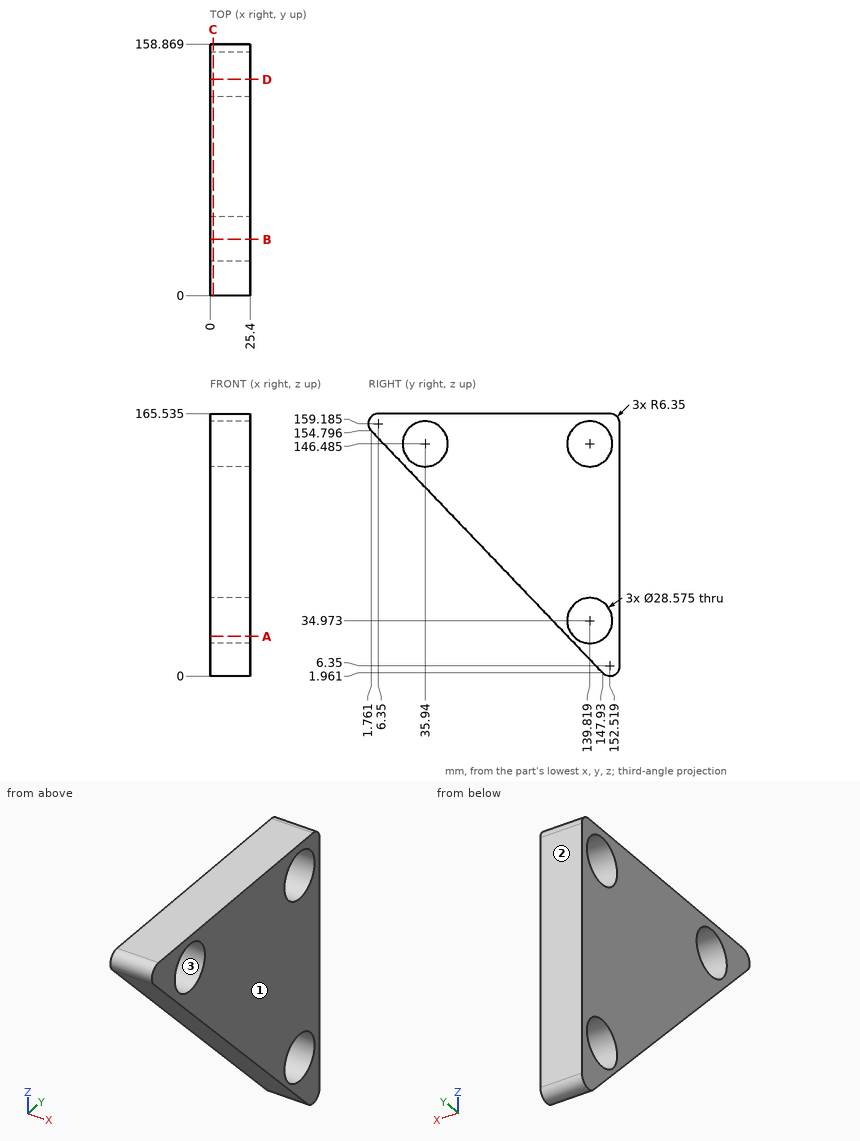
Geometry: see drawing. Coordinates: mm, zero at the bounding-box minimum. Round coordinates to 2 decimals unless told otherwise and drop trailing zeros. Write each loop counter-clockwise with the first axis right and the second up, starting at its lowest first coordinate (ties: lowest second). Pieces come first, ordered by that corner, then holes. Notation, with made-up numbers: M 48,73 L 97,73 A26 cw 97,97 Z; hole C 32.5,57.5 d10. An arc over 180 degrees is marked long. Answer as a JSON object with one key per item and string values. Group by question number.
(1) Section query B-B on y = 35.5. Output: boundary loops of the cut face in (x, z) (1 decimal), then the cut area to 3 significant figures.
(2) First-contact query: pin 1 (4 mm diameter, centred on x = 6.5, z = 50, fed in from -Y) (1 decimal); pin 2 (3 mm diameter, centred on x = 21.5, z = 148, fed in from -Y) (1 decimal); pin 3 (1 mm diameter, centred on x = 20.5, z = 30, fed in from -Y) (1 decimal). Flat tips, straight axial feed; report the tip coordinate or a pass-through.
(3) Section query A-A on z = 25. Output: boundary loops of the cut face in (x, y), then the cut area to 3 significant figures.
(4) Section query D-D on y = 136.5. Output: boundary loops of the cut face in (x, z) (1 decimal).
(5) Section query C-C on x = 2. State how many separate pieces and enclosed holes the cut face has, then the cut area to 3 significant figures.
(6) Mould query, pull axis Y, two halves, no side actions, for the marked faces 1, 2 and 3. Classes: +Y half, -Y half, draft (parallel to the pull), parting line (faces both ways), or undercut.
(7) Ray query, line 1 (Z direction, x = 10.75, y = 130.5) (1 decimal); line 2 (Y direction, x = 3.5, z = 142) (1 decimal); line 3 (Z direction, x = 6.75, y = 34) (1 decimal). Return the intervals inside material, ascending. Write a range as [from, to].
Computed values:
{
 "1": {"outline": "M 0,119.5 L 25.4,119.5 L 25.4,132.2 L 0,132.2 Z; M 0,160.8 L 25.4,160.8 L 25.4,165.5 L 0,165.5 Z", "area": "443 mm^2"},
 "2": {"pin 1": "y = 100.1", "pin 2": "y = 6.8", "pin 3": "y = 120.6"},
 "3": {"outline": "M 0,125.9 L 25.4,125.9 L 25.4,129.59 L 0,129.59 Z; M 0,150.05 L 25.4,150.05 L 25.4,158.87 L 0,158.87 Z", "area": "318 mm^2"},
 "4": {"outline": "M 0,13.9 L 25.4,13.9 L 25.4,21.1 L 0,21.1 Z; M 0,48.9 L 25.4,48.9 L 25.4,132.6 L 0,132.6 Z; M 0,160.4 L 25.4,160.4 L 25.4,165.5 L 0,165.5 Z"},
 "5": {"separate pieces": "1", "enclosed holes": "3", "area": "12,600 mm^2"},
 "6": {"face 1": "draft", "face 2": "+Y half", "face 3": "undercut"},
 "7": {"line 1": "[20.2, 24.1], [45.8, 135.7], [157.3, 165.5]", "line 2": "[14, 22.4], [49.5, 126.3], [153.4, 158.9]", "line 3": "[121.1, 132.3], [160.6, 165.5]"}
}
